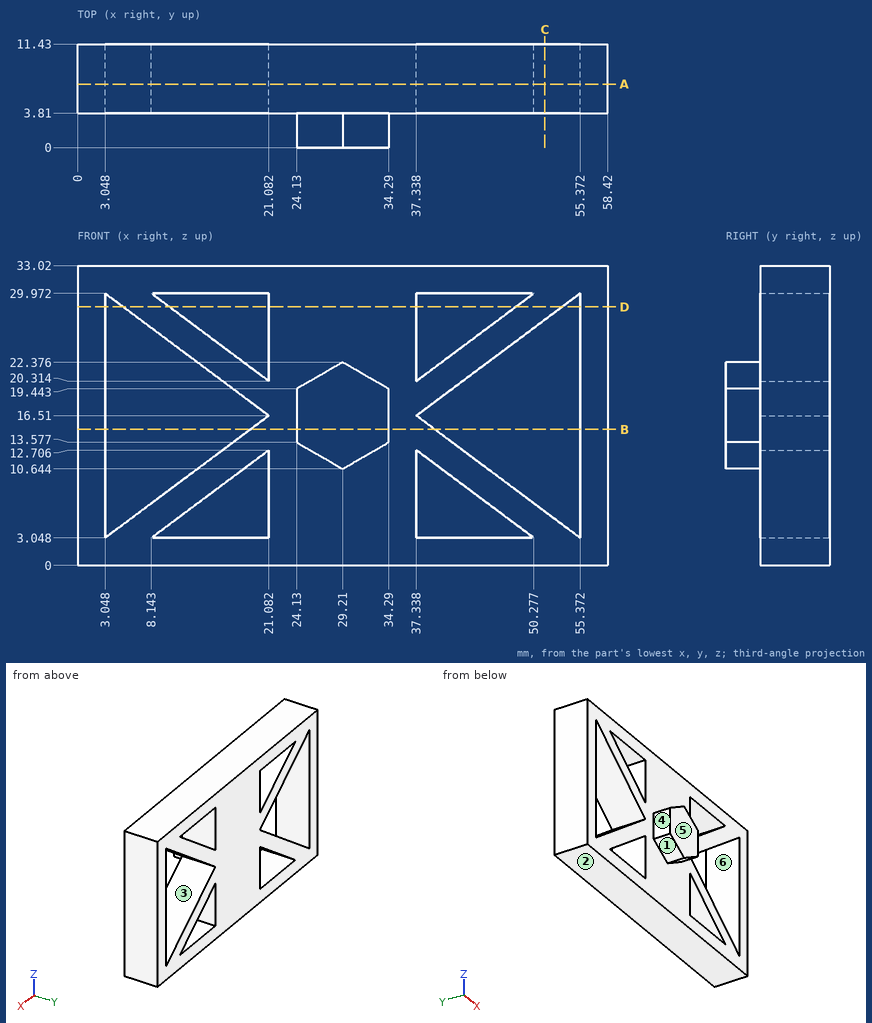
Design review of the part shown in the three views and the two pictorial views. Dimensions are in mm from the part's minimum x, y and z. A direction names the side the tool comes from. Give positions to 0.01 mm unless a question says otherwise; leave off trailing zeros. Loops run counter-clockwise (first coordinate to the right, second up) from the corner with the lowest first, then second, coordinate; pieces in that order, holes last. Notation, with made-up numbers: (16.5, 75) - (42.5, 75) arc R28 cw to (42.5, 97) - close; hole circle Ø1 at (31.5, 40). An arc over 180 degrees is marked (long way). Use CSV: the item, a comma, the result in double quotes. Start each with the question number.
1. Machinability: for the marked faces 4, 5 and 6, which of the approach directions +Z, -Z, +X, -X, +Y, -Y give a long, thin tool a straight path to every point of the face, cutting with its end or side? Answer none if there is none.
2. Draft analysis for pull direction X (two halves, no side actions). For the marked faces 1, 2 and 3, state which applies: released by +X, released by -X, zero draft, split by the parting line, or undercut.
3. Insertion check: P1, Ø1.5, axis at x = 39, y = 7.5, coming from the -Z side; P2, Ø1.9, axis at y = 1.5, z = 17.5, coming from the -X side; P3, Ø6, axis at x = 34.5, z = 8, coming from the -Y side; P4, Ø3, axis at y = 1.5, z = 15.5, coming from the +X side. Each pin has a flat end and moves straight along its axis. Give the tip position at first contact, or say it passes through.
4. Wall thickness on L1, parallel to Z at x = 38.5, y = 9; L2, parallel to Y at x = 54.5, z = 32.5; L3, parallel to Z at x = 55, y = 9.75 (1 decimal): over which ranges is each line inside the solid? List them lowest first.
5. Add section C-C (x = 51.5). State the section outline as (y, z) points, plus the area to 3 significant figures.
6. Add section B-B (z = 15). State the section outline as (x, y) points, plus the area to 3 significant figures.
7. Add section A-A (y = 7). State the section outline as (x, z) points, plus the area to 3 significant figures.
8. Add section D-D (z = 28.5). State the section outline as (x, y) points (1 decimal).
Results found:
1,face 4,"+Z, -Z, -X, -Y"
1,face 5,"+Z, -Z, +X, -X, -Y"
1,face 6,"+Y, -Y"
2,face 1,"released by -X"
2,face 2,"zero draft"
2,face 3,"undercut"
3,P1,"stops at z = 0"
3,P2,"stops at x = 24.13"
3,P3,"stops at y = 3.81"
3,P4,"stops at x = 34.29"
4,L1,"z = 0 to 3.05, 11.84 to 15.64, 17.38 to 21.18, 29.97 to 33.02"
4,L2,"y = 3.81 to 11.43"
4,L3,"z = 0 to 3.3, 29.7 to 33"
5,outline,"(3.81, 0) - (11.43, 0) - (11.43, 5.94) - (3.81, 5.94) - close; (3.81, 27.08) - (11.43, 27.08) - (11.43, 33.02) - (3.81, 33.02) - close"
5,area,"90.5 mm²"
6,outline,"(0, 3.81) - (3.05, 3.81) - (3.05, 11.43) - (0, 11.43) - close; (19.06, 3.81) - (24.13, 3.81) - (24.13, 0) - (34.29, 0) - (34.29, 3.81) - (39.36, 3.81) - (39.36, 11.43) - (19.06, 11.43) - close; (55.37, 3.81) - (58.42, 3.81) - (58.42, 11.43) - (55.37, 11.43) - close"
6,area,"240 mm²"
7,outline,"(0, 0) - (58.42, 0) - (58.42, 33.02) - (0, 33.02) - close; hole (3.05, 3.05) - (21.08, 16.51) - (3.05, 29.97) - close; hole (8.14, 3.05) - (21.08, 3.05) - (21.08, 12.71) - close; hole (8.14, 29.97) - (21.08, 20.31) - (21.08, 29.97) - close; hole (37.34, 3.05) - (50.28, 3.05) - (37.34, 12.71) - close; hole (37.34, 16.51) - (55.37, 3.05) - (55.37, 29.97) - close; hole (37.34, 20.31) - (50.28, 29.97) - (37.34, 29.97) - close"
7,area,"1,190 mm²"
8,outline,"(0, 3.8) - (3, 3.8) - (3, 11.4) - (0, 11.4) - close; (5, 3.8) - (10.1, 3.8) - (10.1, 11.4) - (5, 11.4) - close; (21.1, 3.8) - (37.3, 3.8) - (37.3, 11.4) - (21.1, 11.4) - close; (48.3, 3.8) - (53.4, 3.8) - (53.4, 11.4) - (48.3, 11.4) - close; (55.4, 3.8) - (58.4, 3.8) - (58.4, 11.4) - (55.4, 11.4) - close"
